Drawing for the job (mm, zero at the part's lowest x, y, z). Coordinates: 2 decimals unless noted, no trailing zeros. Order: outer loops, then holes, each group sorted by start corner. A loop starts at its lowest first (then second) coordinate and runs counter-clockwise, first axis right, second up. Notation, with made-up numbers: (0.25, 52) -> (41.25, 52) arc R12 cw to (41.25, 58) -> close; hole circle Ø1 at (-33.5, 12). An arc over 180 degrees is marked (long way). Write each question's results on one line, items separated by ' | '.
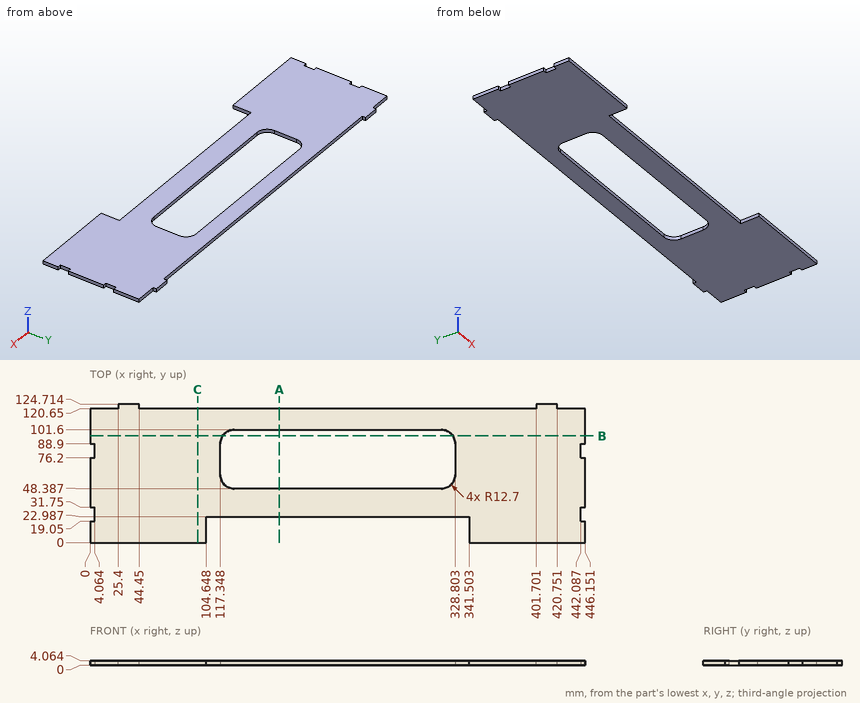
Item 1: Drill centre lines: line 1 (X direction, y = 83, z = 1.05); line 2 (Y direction, x = 267.5, z = 0.9); line 3 (X direction, y = 69, z = 2.5). Where is each one in solid material? Low to high. Write a range as from..to.
Answer:
line 1: x = 4.06..117.35, 328.8..442.09 | line 2: y = 22.99..48.39, 101.6..120.65 | line 3: x = 0..117.35, 328.8..446.15
Item 2: Slice it at C-C, the plane x = 97. List the corners of the cut face in (y, z).
Answer:
outline: (0, 0) -> (120.65, 0) -> (120.65, 4.06) -> (0, 4.06) -> close
Item 3: Slice it at A-A, the plane x = 170.5. List the corners of the cut face in (y, z).
Answer:
outline: (22.99, 0) -> (48.39, 0) -> (48.39, 4.06) -> (22.99, 4.06) -> close; (101.6, 0) -> (120.65, 0) -> (120.65, 4.06) -> (101.6, 4.06) -> close
Item 4: Pin check, flat tips, straight feed: pin 1 (2 mm diameter, centred on x = 433, z = 2, fed in from +Y); pin 2 (2 mm diameter, centred on x = 285, z = 0.5, fed in from -Y); pin 3 (2 mm diameter, centred on y = 80.5, z = 1.5, fed in from -X); pin 4 (1.5 mm diameter, centred on x = 258.5, y = 100, fed in from -Z). Stop position of each tip, or through.
Answer:
pin 1: stops at y = 120.65 | pin 2: stops at y = 22.99 | pin 3: stops at x = 4.06 | pin 4: passes through
Item 5: Slice it at B-B, the plane y = 96. List the corners of the cut face in (x, z), and give its area (3 significant figures).
Answer:
outline: (0, 0) -> (119.52, 0) -> (119.52, 4.06) -> (0, 4.06) -> close; (326.63, 0) -> (446.15, 0) -> (446.15, 4.06) -> (326.63, 4.06) -> close | area: 971 mm^2
